Part print with two shaded views. Sizes in mm from the minimum x, y, z corner. A direction names the side the tool comes from. Round coordinates to 2 decimals unless told otherwise and drop trailing zeros. Loops run counter-clockwise (first coordinate to the right, second up) from the corner with the lowest first, then second, coordinate; pieces in that order, holes last.
(1) Cut at B-B on z = 12. List the corners of the cut face in (x, y).
(2) Cut at C-C on x = 9. List the corners of the cut face in (y, z).
(3) Cut at A-A on y = 28. List the corners of the cut face in (x, z), then the cut area to 3 significant figures.
(4) Tool access for the marked faces 1 and 2: list every direction of +Z, -Z, +X, -X, +Y, -Y with a clear straight run to the whole face (end or side of a thin tool).
(5) Cut at D-D on x = 37. List the corners of the cut face in (y, z), then the cut area to 3 significant figures.
(6) Probe probe 1 along Z at (x, y) = (4, 24); probe 2 along Y at (x, z) = (40.5, 120); probe 3 along Z at (x, y) = (14, 33.5). List the from-to ranges inside material, lowest first.
(7) Flat gauge pins, fed straight in: pin 1 (8 mm diameter, centred on x = 26, z = 146.5, fed in from -Y); pin 2 (10 mm diameter, centred on y = 30.5, z = 22, fed in from -X); pin 3 (20 mm diameter, centred on x = 18.5, y = 16, fed in from -Z); pin 4 (1.8 mm diameter, centred on y = 34, z = 7.5, fed in from +X). Where does each tip first touch, or does it go through?
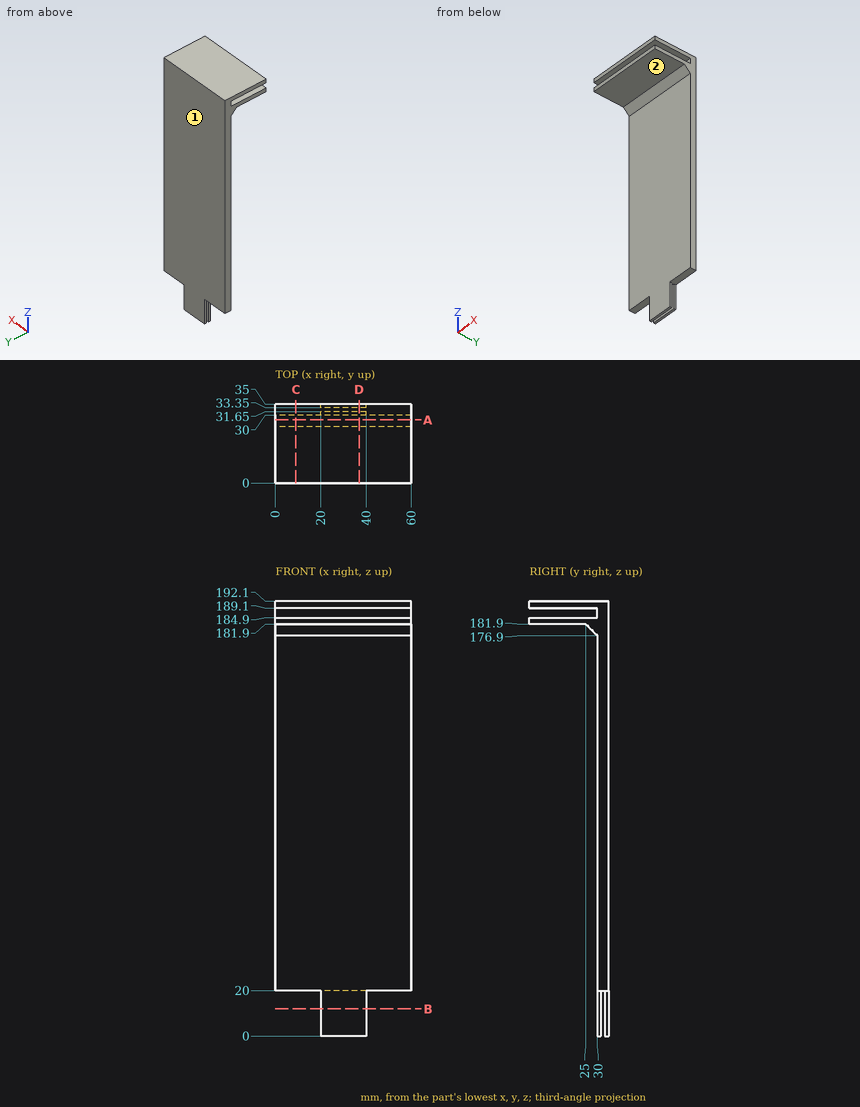
Final values:
1. outline: (20, 30) - (40, 30) - (40, 31.65) - (20, 31.65) - close; (20, 33.35) - (40, 33.35) - (40, 35) - (20, 35) - close
2. outline: (0, 181.9) - (25, 181.9) - (30, 176.9) - (30, 20) - (35, 20) - (35, 192.1) - (0, 192.1) - (0, 189.1) - (30, 189.1) - (30, 184.9) - (0, 184.9) - close
3. outline: (0, 178.9) - (60, 178.9) - (60, 184.9) - (0, 184.9) - close; (0, 189.1) - (60, 189.1) - (60, 192.1) - (0, 192.1) - close
3. area: 540 mm2
4. face 1: +Z, -Z, +X, -X, +Y
4. face 2: -Z, +X, -X, -Y
5. outline: (0, 181.9) - (25, 181.9) - (30, 176.9) - (30, 0) - (31.65, 0) - (31.65, 20) - (33.35, 20) - (33.35, 0) - (35, 0) - (35, 192.1) - (0, 192.1) - (0, 189.1) - (30, 189.1) - (30, 184.9) - (0, 184.9) - close
5. area: 1,120 mm2
6. probe 1: z = 181.9 to 184.9, 189.1 to 192.1
6. probe 2: y = 30 to 35
6. probe 3: z = 20 to 192.1
7. pin 1: stops at y = 30
7. pin 2: stops at x = 0
7. pin 3: stops at z = 180.9
7. pin 4: stops at x = 40
